Verification items for the finished model (mm, model axes). A direction names the side the tool comes from. Coordinates: 2 decimals unless noted, no trailing zeros. Loops run counter-clockwise (first coordinate to the right, second up) from the corner with the lowest first, then second, coordinate; pieces in that order, holes last.
Q1. Sectioned sample at B-B (z = 6.25). Count the separate pieces of the cut face and the enclosed holes in it, then the cut area to 3 significant figures.
Q2. Sectioned sample at A-A (y = 2.5). Enter the section's corners in (x, z).
Q3. Access from +Z, -Z, +X, -X, +Y, -Y to the whole of each face (thin tool, end or side, straight path). Record for faces 1 (the face through (-2, 24.015, 4)), 2 (the face through (12.577, -4, 4)), 3 (the face through (-1, 100.015, 6)).
Q4. Go/stop test with flat-tipped pins: P1, Ø4, axis at x = 5, y = 217.5, coming from the +Z side; P2, Ø4, axis at y = 87.5, z = 4.5, coming from the +X side; P3, Ø1.1, axis at y = 96.5, z = 6.5, coming from the -X side. Record where each tip stops, or that it passes through.
Q5. Material ranges on probe 1 along Y at (x, z) = (-14, 1); probe 2 along Y at (x, z) = (22, 5); probe 3 along Y at (x, z) = (35.5, 7.25), recorded low to high.
Q6. Mould release check, pull along Y, two halves, no side actions. Record for faces 4 (the face through (-19.423, -4, 4)), 5 (the face through (1, 96, 4)), 6 (the face through (9, -31.985, 4)), 7 (the face through (15.577, 116, 4)): +Y half, -Y half, draft (parallel to the pull), parting line (faces both ways), or undercut.
Q7. Sectioned sample at D-D (y = 190.5). Enter the section's corners in (x, z), then the cut area to 3 significant figures.
```python
from build123d import *

# Parameters (mm, degrees)
ESQUISSE1_W             = 10
ESQUISSE1_H             = 24
BOSS_EXTRU_1_DEPTH      = 8
ESQUISSE2_W             = 53.566329485
ESQUISSE2_H             = 7.982626226
ESQUISSE2_W_2           = 58
ESQUISSE2_H_2           = 8
ENL_V_MAT_EXTRU_1_DEPTH = 4
ESQUISSE3_R             = 0.5
ESQUISSE3_R_2           = 1
ENL_V_MAT_EXTRU_2_DEPTH = 4


with BuildPart() as part:
    # Esquisse1 → Boss.-Extru.1 (new body)
    with BuildSketch(Plane.XY):
        with BuildLine():
            Line((30.577007139, 186.135890651), (30.577007139, 224.014570308))
            Line((30.577007139, 224.014570308), (-19.422992861, 224.014570308))
            Line((-19.422992861, 224.014570308), (-19.422992861, 208.031944082))
            Line((-19.422992861, 208.031944082), (15.577007139, 208.031944082))
            Line((15.577007139, 208.031944082), (15.577007139, 184.014570308))
            Line((15.577007139, 184.014570308), (-19.422992861, 184.014570308))
            Line((-19.422992861, 184.014570308), (-19.422992861, 168.014570308))
            Line((-19.422992861, 168.014570308), (15.577007139, 168.014570308))
            Line((15.577007139, 168.014570308), (15.577007139, 144.014570308))
            Line((15.577007139, 144.014570308), (-19.422992861, 144.014570308))
            Line((-19.422992861, 144.014570308), (-19.422992861, 128.014570308))
            Line((-19.422992861, 128.014570308), (15.577007139, 128.014570308))
            Line((15.577007139, 128.014570308), (15.577007139, 104.014570308))
            Line((15.577007139, 104.014570308), (-19.422992861, 104.014570308))
            Line((-19.422992861, 104.014570308), (-19.422992861, 88.014570308))
            Line((-19.422992861, 88.014570308), (15.577007139, 88.014570308))
            Line((15.577007139, 88.014570308), (15.577007139, 64.014570308))
            Line((15.577007139, 64.014570308), (-19.422992861, 64.014570308))
            Line((-19.422992861, 64.014570308), (-19.422992861, 48.014570308))
            Line((-19.422992861, 48.014570308), (15.577007139, 48.014570308))
            Line((15.577007139, 48.014570308), (15.577007139, 24.014570308))
            Line((15.577007139, 24.014570308), (-19.422992861, 24.014570308))
            Line((-19.422992861, 24.014570308), (-19.422992861, -31.985429692))
            Line((-19.422992861, -31.985429692), (30.577007139, -31.985429692))
            Line((30.577007139, -31.985429692), (38.577007139, -31.985429692))
            Line((38.577007139, -31.985429692), (38.577007139, 18.014570308))
            Line((38.577007139, 18.014570308), (32.698327483, 18.014570308))
            ThreePointArc((32.698327483, 18.014570308), (30.577007139, 18.014570308), (30.577007139, 20.135890651))
            Line((30.577007139, 20.135890651), (30.577007139, 131.893249964))
            ThreePointArc((30.577007139, 131.893249964), (30.577007139, 134.014570308), (32.698327483, 134.014570308))
            Line((32.698327483, 134.014570308), (38.577007139, 134.014570308))
            Line((38.577007139, 134.014570308), (38.577007139, 184.014570308))
            Line((38.577007139, 184.014570308), (32.698327483, 184.014570308))
            ThreePointArc((32.698327483, 184.014570308), (30.577007139, 184.014570308), (30.577007139, 186.135890651))
        make_face()
        with Locations((17.577007139, -3.985429692)):
            Rectangle(ESQUISSE1_W, ESQUISSE1_H, mode=Mode.SUBTRACT)
    extrude(amount=BOSS_EXTRU_1_DEPTH)

    # Esquisse2 → Enlèv. mat.-Extru.1 (cut)
    with BuildSketch(Plane.XY.offset(8)):
        with BuildLine():
            Line((-19.422992861, 140.014570308), (18.455686796, 140.014570308))
            ThreePointArc((18.455686796, 140.014570308), (20.577007139, 140.014570308), (20.577007139, 137.893249964))
            Line((20.577007139, 137.893249964), (20.577007139, 134.135890651))
            ThreePointArc((20.577007139, 134.135890651), (20.577007139, 132.014570308), (18.455686796, 132.014570308))
            Line((18.455686796, 132.014570308), (-19.422992861, 132.014570308))
            Line((-19.422992861, 132.014570308), (-19.422992861, 140.014570308))
        make_face()
        with BuildLine():
            Line((-19.422992861, 100.014570308), (18.455686796, 100.014570308))
            ThreePointArc((18.455686796, 100.014570308), (20.577007139, 100.014570308), (20.577007139, 97.893249964))
            Line((20.577007139, 97.893249964), (20.577007139, 94.135890651))
            ThreePointArc((20.577007139, 94.135890651), (20.577007139, 92.014570308), (18.455686796, 92.014570308))
            Line((18.455686796, 92.014570308), (-19.422992861, 92.014570308))
            Line((-19.422992861, 92.014570308), (-19.422992861, 100.014570308))
        make_face()
        with BuildLine():
            Line((-19.422992861, 60.014570308), (18.455686796, 60.014570308))
            ThreePointArc((18.455686796, 60.014570308), (20.577007139, 60.014570308), (20.577007139, 57.893249964))
            Line((20.577007139, 57.893249964), (20.577007139, 54.135890651))
            ThreePointArc((20.577007139, 54.135890651), (20.577007139, 52.014570308), (18.455686796, 52.014570308))
            Line((18.455686796, 52.014570308), (-19.422992861, 52.014570308))
            Line((-19.422992861, 52.014570308), (-19.422992861, 60.014570308))
        make_face()
        with BuildLine():
            Line((-19.422992861, 180.014570308), (28.510535818, 180.014570308))
            ThreePointArc((28.510535818, 180.014570308), (30.446580511, 179.833376068), (30.577007139, 177.893249964))
            Line((30.577007139, 177.893249964), (30.577007139, 174.135890651))
            ThreePointArc((30.577007139, 174.135890651), (30.446580511, 172.195764547), (28.510535818, 172.014570308))
            Line((28.510535818, 172.014570308), (-19.422992861, 172.014570308))
            Line((-19.422992861, 172.014570308), (-19.422992861, 180.014570308))
        make_face()
        with BuildLine():
            Line((-19.422992861, 20.014570308), (18.455686796, 20.014570308))
            ThreePointArc((18.455686796, 20.014570308), (20.577007139, 20.014570308), (20.577007139, 17.893249964))
            Line((20.577007139, 17.893249964), (20.577007139, 14.135890651))
            ThreePointArc((20.577007139, 14.135890651), (20.577007139, 12.014570308), (18.455686796, 12.014570308))
            Line((18.455686796, 12.014570308), (-19.422992861, 12.014570308))
            Line((-19.422992861, 12.014570308), (-19.422992861, 20.014570308))
        make_face()
        with Locations((7.360171881, 216.023257195)):
            Rectangle(ESQUISSE2_W, ESQUISSE2_H)
        with Locations((9.577007139, -23.985429692)):
            Rectangle(ESQUISSE2_W_2, ESQUISSE2_H_2)
    extrude(amount=-ENL_V_MAT_EXTRU_1_DEPTH, mode=Mode.SUBTRACT)

    # Esquisse3 → Enlèv. mat.-Extru.2 (cut)
    with BuildSketch(Plane.XY.offset(4)):
        with Locations((15.577007139, 216.023257195)):
            Circle(ESQUISSE3_R)
        with Locations((24.077007139, -23.985429692)):
            Circle(ESQUISSE3_R_2)
        with Locations(Location((-4.922992861, -23.985429692, 0), (0, 0, 180))):
            Circle(ESQUISSE3_R_2)
    extrude(amount=-ENL_V_MAT_EXTRU_2_DEPTH, mode=Mode.SUBTRACT)


solid = part.part
```
Geometry check:
1. separate pieces: 3
1. enclosed holes: 1
1. area: 6,600 mm2
2. outline: (-19.42, 0) - (12.58, 0) - (12.58, 8) - (-19.42, 8) - close; (22.58, 0) - (38.58, 0) - (38.58, 8) - (22.58, 8) - close
3. face 1: +Z, -Z, -X
3. face 2: +Z, -Z
3. face 3: +Z, -X
4. P1: stops at z = 4
4. P2: stops at x = 30.58
4. P3: stops at x = 20.58
5. probe 1: y = -31.99 to 24.01, 48.01 to 64.01, 88.01 to 104.01, 128.01 to 144.01, 168.01 to 184.01, 208.03 to 224.01
5. probe 2: y = -31.99 to -27.99, -19.99 to -15.99, 8.01 to 172.01, 180.01 to 212.03, 220.01 to 224.01
5. probe 3: y = -31.99 to -27.99, -19.99 to 18.01, 134.01 to 184.01
6. face 4: draft
6. face 5: undercut
6. face 6: -Y half
6. face 7: undercut
7. outline: (15.58, 0) - (30.58, 0) - (30.58, 8) - (15.58, 8) - close
7. area: 120 mm2
